Part model, mm, in its own coordinate system. A direction names the side the tool comes from. Give positions to 0.01 mm unless a question says otherwise; leave off trailing zeros. Write each loop counter-clockwise with the first axis right and the second up, starting at its lowest first coordinate (ties: lowest second). Pieces come first, ordered by that corner, then holes. Notation, with made-up numbers: (14.25, 51.25) - (44.25, 51.25) arc R23 ccw to (44.25, 78.25) - close; hole circle Ø8 at (26.25, 69). An arc over 180 degrees is marked (long way). Answer as a JSON object with one key per item and string values. Group by question number.
```python
from build123d import *

# Parameters (mm, degrees)
SKETCH1_W           = 127
SKETCH1_H           = 177.8
BOSS_EXTRUDE1_DEPTH = 6.35
CUT_EXTRUDE1_DEPTH  = 219.591313871
SKETCH3_R           = 1.905
CUT_EXTRUDE2_DEPTH  = 219.591313871


with BuildPart() as part:
    # Sketch1 → Boss-Extrude1 (new body)
    with BuildSketch(Plane(origin=(0, 0, 0), x_dir=(1, 0, 0), z_dir=(0, 1, 0))):
        with Locations((63.5, 88.9)):
            Rectangle(SKETCH1_W, SKETCH1_H)
    extrude(amount=BOSS_EXTRUDE1_DEPTH)

    # Sketch2 → Cut-Extrude1 (cut, through all)
    with BuildSketch(Plane(origin=(0, 6.35, 0), x_dir=(1, 0, 0), z_dir=(0, 1, 0))):
        Polygon((114.554, 167.411684877), (12.446, 167.411684877), (12.446, 12.446), (89.408, 12.446), (114.554, 37.592), align=None)
    extrude(amount=-CUT_EXTRUDE1_DEPTH, mode=Mode.SUBTRACT)

    # Sketch3 → Cut-Extrude2 (cut, through all)
    with BuildSketch(Plane(origin=(0, 6.35, 0), x_dir=(1, 0, 0), z_dir=(0, 1, 0))):
        with Locations(Location((6.35, 171.45, 0), (0, 0, 270))):
            Circle(SKETCH3_R)
        with Locations(Location((6.35, 6.35, 0), (0, 0, 90))):
            Circle(SKETCH3_R)
        with Locations(Location((120.65, 6.35, 0), (0, 0, 270))):
            Circle(SKETCH3_R)
        with Locations(Location((120.65, 171.45, 0), (0, 0, 90))):
            Circle(SKETCH3_R)
    extrude(amount=-CUT_EXTRUDE2_DEPTH, mode=Mode.SUBTRACT)


solid = part.part
```
1) Drop a flat-ended pin along its axis: P1, Ø3.5, axis at x = 6.35, z = -171.45, coming from the -Y side. Give the stop position or say it passes through.
2) Which spindle directions (+Z, -Z, +X, -X, +Y, -Y) get a long thin tool onto all of the face, cutting with end or side? Do faces 4 (the flat face through (0, 3, -88)), 5 (the flat face through (12.446, 3, -91)). Say none if no direction does.
3) Mould opens along Z. For faces 1 (the flat face through (119, 0, -90)), 2 (the cylindrical face through (8.2, 3.2, -5.9)), 3 (the flat face through (63, 3, 0)) say: pulls with the +Z half, pulls with the -Z half, needs draft (parallel to the pull), parting line crosses it, or undercut.
4) Band-saw the part on B-B (x = 120.65). List the corners of the cut face in (y, z) (3 decimals).
5) Band-saw the part on A-A (z = -44). List the corners of the cut face in (x, y), plus the area to 3 significant figures.
6) Band-saw the part on C-C (y = 1.25). List the corners of the cut face in (x, z) (3 decimals), plus the area to 3 significant figures.
7) Band-saw the part on D-D (z = -171.45). List the corners of the cut face in (x, y) (3 decimals), plus the area to 3 significant figures.
8) Probe line 1 (X direction, y = 4.25, z = -6.35) (3 decimals); line 2 (Z direction, x = 76, y = 4.25); line 3 (X direction, y = 1.5, z = -81). List the from-to ranges inside material, lowest first.
Verdict:
{
 "1": {"P1": "through"},
 "2": {"face 4": "+Z, -Z, -X, +Y, -Y", "face 5": "+Y, -Y"},
 "3": {"face 1": "needs draft", "face 2": "undercut", "face 3": "pulls with the +Z half"},
 "4": {"outline": "(0, -177.8) - (6.35, -177.8) - (6.35, -173.355) - (0, -173.355) - close; (0, -169.545) - (6.35, -169.545) - (6.35, -8.255) - (0, -8.255) - close; (0, -4.445) - (6.35, -4.445) - (6.35, 0) - (0, 0) - close"},
 "5": {"outline": "(0, 0) - (12.45, 0) - (12.45, 6.35) - (0, 6.35) - close; (114.55, 0) - (127, 0) - (127, 6.35) - (114.55, 6.35) - close", "area": "158 mm2"},
 "6": {"outline": "(0, -177.8) - (127, -177.8) - (127, 0) - (0, 0) - close; hole circle Ø3.81 at (6.35, -171.45); hole circle Ø3.81 at (6.35, -6.35); hole (12.446, -167.412) - (114.554, -167.412) - (114.554, -37.592) - (89.408, -12.446) - (12.446, -12.446) - close; hole circle Ø3.81 at (120.65, -171.45); hole circle Ø3.81 at (120.65, -6.35)", "area": "7,030 mm2"},
 "7": {"outline": "(0, 0) - (4.445, 0) - (4.445, 6.35) - (0, 6.35) - close; (8.255, 0) - (118.745, 0) - (118.745, 6.35) - (8.255, 6.35) - close; (122.555, 0) - (127, 0) - (127, 6.35) - (122.555, 6.35) - close", "area": "758 mm2"},
 "8": {"line 1": "0 to 4.445, 8.255 to 118.745, 122.555 to 127", "line 2": "-177.8 to -167.41, -12.45 to 0", "line 3": "0 to 12.45, 114.55 to 127"}
}
